The listing builds one solid part. Answer for the finished solid, in the listing's coordinates (mm). A direction names the side the tool comes from. Give positions to 0.01 mm unless a question says otherwise; leave off trailing zeros. Order: outer loops, then holes, each group sorted by start corner. A loop starts at its lowest first (then second) coordinate and runs counter-clockwise, first axis right, second up. Notation, with made-up numbers: (-39, 75) - (11, 75) arc R24 ccw to (11, 103) - close; hole circle Ø11 at (43.5, 71). An arc over 180 degrees is marked (long way). Answer in a Markdown table with one row per item. Add a question column.
```python
from build123d import *

# Parameters (mm, degrees)
BOSS_EXTRUDE1_DEPTH = 3
FILLET1_R           = 3
SKETCH2_R           = 10
BOSS_EXTRUDE3_DEPTH = 70
SKETCH4_R           = 2.5
CUT_EXTRUDE2_DEPTH  = 70
SKETCH7_R           = 3.25
CUT_EXTRUDE3_DEPTH  = 38
FILLET3_R           = 4
SKETCH8_R           = 5
CUT_EXTRUDE4_DEPTH  = 70
SKETCH10_W          = 35
SKETCH10_H          = 35
BOSS_EXTRUDE5_DEPTH = 3
FILLET5_R           = 3
SKETCH11_R          = 2.5
BOSS_EXTRUDE6_DEPTH = 10
FILLET6_R           = 4


with BuildPart() as part:
    # Sketch1 → Boss-Extrude1 (new body)
    with BuildSketch(Plane(origin=(0, 0, 0), x_dir=(1, 0, 0), z_dir=(0, 1, 0))):
        with BuildLine():
            ThreePointArc((0, 30), (21.213203436, 21.213203436), (30, 0))
            Line((30, 0), (40, 0))
            ThreePointArc((40, 0), (48.786796564, 21.213203436), (70, 30))
            Line((70, 30), (70, 40))
            ThreePointArc((70, 40), (48.786796564, 48.786796564), (40, 70))
            Line((40, 70), (30, 70))
            ThreePointArc((30, 70), (21.213203436, 48.786796564), (0, 40))
            Line((0, 40), (0, 30))
        make_face()
    extrude(amount=BOSS_EXTRUDE1_DEPTH)

    # Fillet1
    fillet1_edges = [part.edges().sort_by_distance(p)[0] for p in [
        (70, 1.5, -40),
        (70, 1.5, -30),
        (40, 1.5, 0),
        (30, 1.5, 0),
        (0, 1.5, -30),
        (0, 1.5, -40),
        (30, 1.5, -70),
        (40, 1.5, -70),
    ]]
    fillet(fillet1_edges, radius=FILLET1_R)

    # Sketch2 → Boss-Extrude3 (add)
    with BuildSketch(Plane(origin=(0, 3, 0), x_dir=(1, 0, 0), z_dir=(0, 1, 0))):
        with Locations(Location((35, 35, 0), (0, 0, 270))):
            Circle(SKETCH2_R)
    extrude(amount=BOSS_EXTRUDE3_DEPTH)

    # Sketch4 → Cut-Extrude2 (cut)
    with BuildSketch(Plane(origin=(70, 0, 0), x_dir=(0, 0, -1), z_dir=(1, 0, 0))):
        with Locations((35, 65)):
            Circle(SKETCH4_R)
    extrude(amount=-CUT_EXTRUDE2_DEPTH, mode=Mode.SUBTRACT)

    # Sketch7 → Cut-Extrude3 (cut)
    with BuildSketch(Plane(origin=(70, 0, 0), x_dir=(0, 0, -1), z_dir=(1, 0, 0))):
        with Locations((35, 65)):
            Circle(SKETCH7_R)
    extrude(amount=-CUT_EXTRUDE3_DEPTH, mode=Mode.SUBTRACT)

    # Fillet3
    fillet3_edges = [part.edges().sort_by_distance(p)[0] for p in [
        (35, 73, -45),
    ]]
    fillet(fillet3_edges, radius=FILLET3_R)

    # Sketch8 → Cut-Extrude4 (cut)
    with BuildSketch(Plane(origin=(0, 73, 0), x_dir=(1, 0, 0), z_dir=(0, 1, 0))):
        with Locations((45, 35)):
            Circle(SKETCH8_R)
    extrude(amount=-CUT_EXTRUDE4_DEPTH, mode=Mode.SUBTRACT)

    # Sketch10 → Boss-Extrude5 (add)
    with BuildSketch(Plane(origin=(0, 3, 0), x_dir=(1, 0, 0), z_dir=(0, 1, 0))):
        with Locations((52.5, 52.5)):
            Rectangle(SKETCH10_W, SKETCH10_H)
    extrude(amount=-BOSS_EXTRUDE5_DEPTH)

    # Fillet5
    fillet5_edges = [part.edges().sort_by_distance(p)[0] for p in [
        (70, 1.5, -70),
    ]]
    fillet(fillet5_edges, radius=FILLET5_R)

    # Sketch11 → Boss-Extrude6 (add)
    with BuildSketch(Plane(origin=(0, 3, 0), x_dir=(1, 0, 0), z_dir=(0, 1, 0))):
        with Locations(Location((67, 67, 0), (0, 0, 270))):
            Circle(SKETCH11_R)
        with Locations(Location((47.5, 47.5, 0), (0, 0, 270))):
            Circle(SKETCH11_R)
    extrude(amount=BOSS_EXTRUDE6_DEPTH)

    # Fillet6
    # the kernel refuses this fillet: 4 mm, written as the material it adds along each edge
    with BuildSketch(Plane(origin=(35, 3, -35), x_dir=(0.9999950652018581, 0, -0.0031415874858794265), z_dir=(0.0031415874858794265, 0, 0.9999950652018581))) as fillet6_piece_1_section:
        with BuildLine():
            CenterArc((10 + FILLET6_R, FILLET6_R), FILLET6_R, 180, 90)
            Line((10, FILLET6_R), (10, 0))
            Line((10, 0), (10 + FILLET6_R, 0))
        make_face()
    fillet6_piece_1 = revolve(axis=Axis((35, 3, -35), (0, 1, 0)), revolution_arc=359.64, mode=Mode.PRIVATE)
    fillet6_piece_1 = fillet6_piece_1 - Plane(origin=(45, 4.127744663, -35), x_dir=(1, 0, 0), z_dir=(0, 1, 0)) * Cylinder(5, 56, mode=Mode.PRIVATE)
    add(fillet6_piece_1)


solid = part.part
```
(1) Straight lines are drawn through the part: line 1 (Y direction, x = 29, z = -35); line 2 (Y direction, x = 58, z = -55.5); line 3 (Z direction, x = 39, y = 65). For each, find the intervals that lie inside material, in ascending order.
(2) Find section D-D, the plane x = 63. Write down the section's boundary in (y, z).
(3) For faces 1 (the face through (25, 38, -35)), 2 (the face through (21.418, 1.479, -48.994)), determine the directions among +Z, -Z, +X, -X, +Y, -Y from which every point of the face is accessible in a straight line to the end or side of a thin tool.
(4) The mould has two halves that part along Y. Classify faces 3 (the face through (32, 63, -37)), 4 (the face through (69.195, 1.521, -30.818)), 5 (the face through (48, 13, -48)): +Y half, -Y half, draft (parallel to the pull), parting line (faces both ways), or undercut.
(5) Find section B-B, the plane x = 35. Write down the section's boundary in (y, z), plus the area to 3 significant figures.
(6) Find section A-A, the plane z = -35. Write down the section's boundary in (x, y).
(7) Find section C-C, the plane z = -52. Write down the section's boundary in (x, y).
(8) Each of these flat-tipped pins is pushed along its axis until it touches: P1, Ø4, axis at x = 67, z = -66.5, coming from the +Y side; P2, Ø9, axis at x = 45, z = -35, coming from the +Y side; P3, Ø10.5, axis at y = 65, z = -35, coming from the +X side. Where does it stop, or does it pass through?
Answer key:
| question | item | result |
|---|---|---|
| 1 | line 1 | 0 to 62.5, 67.5 to 73 |
| 1 | line 2 | 0 to 3 |
| 1 | line 3 | -44.17 to -38.25, -31.75 to -25.83 |
| 2 | outline | (0, -70) - (3, -70) - (3, -29.17) - (0, -29.17) - close |
| 3 | face 1 | +Y |
| 3 | face 2 | -Z, -X, +Y, -Y |
| 4 | face 3 | undercut |
| 4 | face 4 | draft |
| 4 | face 5 | +Y half |
| 5 | outline | (0, -70) - (3, -70) - (3, -49) arc R4 cw to (7, -45) - (69, -45) arc R4 ccw to (73, -41) - (73, -29) arc R4 ccw to (69, -25) - (7, -25) arc R4 cw to (3, -21) - (3, 0) - (0, 0) - close; hole circle Ø6.5 at (65, -35) |
| 5 | area | 1,580 mm² |
| 6 | outline | (0, 0) - (70, 0) - (70, 3) - (40, 3) - (40, 61.75) - (32, 61.75) - (32, 62.5) - (25, 62.5) - (25, 7) arc R4 cw to (21, 3) - (0, 3) - close; (25, 67.5) - (32, 67.5) - (32, 68.25) - (40, 68.25) - (40, 73) - (29, 73) arc R4 ccw to (25, 69) - close |
| 7 | outline | (24, 0) - (70, 0) - (70, 3) - (24, 3) - close |
| 8 | P1 | y = 13 |
| 8 | P2 | y = 3 |
| 8 | P3 | x = 43.75 |
